Geometry: final body of the model. Coordinates: model frame, mm. Face numbers are marked on the shaded views. A direction names the side the tool comes from. Give positions to 0.01 mm unless a question says otherwise; leave off trailing zeros. Loops run counter-clockwise (first coordinate to the right, second up) from the corner with the lowest first, then second, coordinate; pieces in that order, holes last.
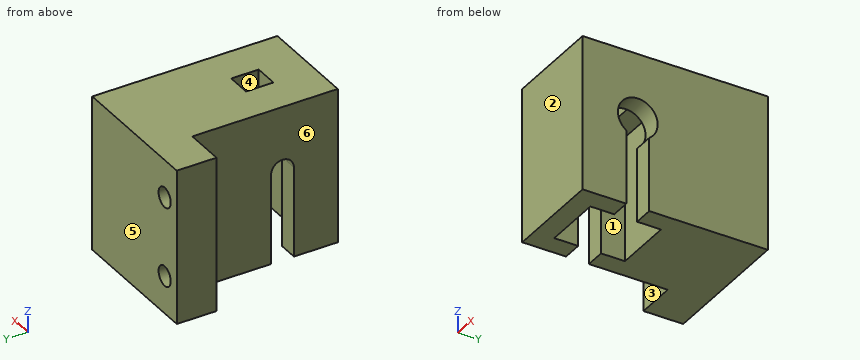
from build123d import *

# Parameters (mm, degrees)
SKETCH1_W           = 31.6
SKETCH1_H           = 35.300000012
SKETCH1_W_2         = 18.9
SKETCH1_H_2         = 22.600000012
BOSS_EXTRUDE1_DEPTH = 40
SKETCH2_W           = 31.6
SKETCH2_H           = 35.300000012
SKETCH2_W_2         = 18.9
SKETCH2_H_2         = 22.600000012
BOSS_EXTRUDE2_DEPTH = 9.525
SKETCH3_W           = 7.74908697
SKETCH3_H           = 8.788598638
CUT_EXTRUDE1_DEPTH  = 12.7
CUT_EXTRUDE2_DEPTH  = 31.75
SKETCH6_W           = 31.6
SKETCH6_H           = 49.525
BOSS_EXTRUDE3_DEPTH = 11.176
BOSS_EXTRUDE4_START = -44.45
SKETCH7_W           = 49.525
SKETCH7_H           = 6.35
BOSS_EXTRUDE4_DEPTH = 57.15
SKETCH8_R           = 3.175
CUT_EXTRUDE3_DEPTH  = 6.35
SKETCH9_W           = 12.85
SKETCH9_H           = 49.525
CUT_EXTRUDE4_DEPTH  = 6.35
SKETCH11_R          = 3.429
SKETCH11_W          = 12.85
SKETCH11_H          = 49.525
CUT_EXTRUDE5_DEPTH  = 6.35
SKETCH12_R          = 6.35
CUT_EXTRUDE6_DEPTH  = 6.35
SKETCH13_W          = 44.3
SKETCH13_H          = 49.525
SKETCH13_R          = 3.175
BOSS_EXTRUDE5_DEPTH = 12.7
SKETCH14_W          = 12.7
SKETCH14_H          = 49.525
SKETCH14_R          = 3.175
CUT_EXTRUDE7_DEPTH  = 6.35


with BuildPart() as part:
    # Sketch1 → Boss-Extrude1 (new body)
    with BuildSketch(Plane.XY):
        Rectangle(SKETCH1_W, SKETCH1_H)
        Rectangle(SKETCH1_W_2, SKETCH1_H_2, mode=Mode.SUBTRACT)
    extrude(amount=BOSS_EXTRUDE1_DEPTH)

    # Sketch2 → Boss-Extrude2 (add)
    # profile 1 of 2: a face of its own
    with BuildSketch(Plane.XY.offset(40)):
        Rectangle(SKETCH2_W, SKETCH2_H)
        Rectangle(SKETCH2_W_2, SKETCH2_H_2, mode=Mode.SUBTRACT)
    # profile 2 of 2: a face of its own
    with BuildSketch(Plane.XY.offset(40)):
        Rectangle(SKETCH2_W_2, SKETCH2_H_2)
    extrude(amount=BOSS_EXTRUDE2_DEPTH)

    # Sketch3 → Cut-Extrude1 (cut)
    with BuildSketch(Plane(origin=(0, 0, 40), x_dir=(-1, 0, 0), z_dir=(0, 0, -1))):
        Rectangle(SKETCH3_W, SKETCH3_H)
    extrude(amount=-CUT_EXTRUDE1_DEPTH, mode=Mode.SUBTRACT)

    # Sketch5 → Cut-Extrude2 (cut)
    with BuildSketch(Plane(origin=(15.8, 0, 0), x_dir=(0, 0, -1), z_dir=(1, 0, 0))):
        with BuildLine():
            Line((-28.827575985, 3.65), (0, 3.65))
            Line((0, 3.65), (0, -3.65))
            Line((0, -3.65), (-28.827575985, -3.65))
            ThreePointArc((-28.827575985, -3.65), (-32.477575985, 0), (-28.827575985, 3.65))
        make_face()
    extrude(amount=-CUT_EXTRUDE2_DEPTH, mode=Mode.SUBTRACT)

    # Sketch6 → Boss-Extrude3 (add)
    with BuildSketch(Plane(origin=(0, 17.650000006, 0), x_dir=(1, 0, 0), z_dir=(0, 1, 0))):
        with Locations((0, -24.7625)):
            Rectangle(SKETCH6_W, SKETCH6_H)
    extrude(amount=BOSS_EXTRUDE3_DEPTH)

    # Sketch7 → Boss-Extrude4 (add)
    with BuildSketch(Plane(origin=(15.8, 0, 0), x_dir=(0, 0, -1), z_dir=(1, 0, 0)).offset(BOSS_EXTRUDE4_START)):
        with Locations((-24.7625, 25.651000006)):
            Rectangle(SKETCH7_W, SKETCH7_H)
    boss_extrude4 = extrude(amount=BOSS_EXTRUDE4_DEPTH)

    # Sketch8 → Cut-Extrude3 (cut)
    with BuildSketch(Plane.XZ.offset(-22.476000006)):
        with Locations(Location((-22.225, 24.7625, 0), (0, 0, 270))):
            Circle(SKETCH8_R)
        with Locations(Location((22.15, 37.434572452, 0), (0, 0, 270))):
            Circle(SKETCH8_R)
        with Locations(Location((22.15, 12.034572452, 0), (0, 0, 270))):
            Circle(SKETCH8_R)
    extrude(amount=-CUT_EXTRUDE3_DEPTH, mode=Mode.SUBTRACT)

    # Sketch9 → Cut-Extrude4 (cut)
    with BuildSketch(Plane.XZ.offset(-22.476000006)):
        with Locations((-22.225, 24.7625)):
            Rectangle(SKETCH9_W, SKETCH9_H)
    extrude(amount=-CUT_EXTRUDE4_DEPTH, mode=Mode.SUBTRACT)

    # Mirror1: Boss-Extrude4 across plane
    add(boss_extrude4.mirror(Plane(origin=(0, 0, 0), x_dir=(0, 0, 1), z_dir=(1, 0, 0))))

    # Sketch11 → Cut-Extrude5 (cut)
    with BuildSketch(Plane(origin=(0, 28.826000006, 0), x_dir=(1, 0, 0), z_dir=(0, 1, 0))):
        with Locations(Location((-22.15, -37.4625, 0), (0, 0, 270))):
            Circle(SKETCH11_R)
        with Locations(Location((-22.15, -12.0625, 0), (0, 0, 270))):
            Circle(SKETCH11_R)
        with Locations((22.225, -24.7625)):
            Rectangle(SKETCH11_W, SKETCH11_H)
    extrude(amount=-CUT_EXTRUDE5_DEPTH, mode=Mode.SUBTRACT)

    # Sketch12 → Cut-Extrude6 (cut)
    with BuildSketch(Plane(origin=(15.8, 0, 0), x_dir=(0, 0, -1), z_dir=(1, 0, 0))):
        with Locations((-28.827575985, 0)):
            Circle(SKETCH12_R)
    extrude(amount=-CUT_EXTRUDE6_DEPTH, mode=Mode.SUBTRACT)

    # Sketch13 → Boss-Extrude5 (add)
    with BuildSketch(Plane(origin=(0, 28.826000006, 0), x_dir=(1, 0, 0), z_dir=(0, 1, 0))):
        with Locations((-6.35, -24.7625)):
            Rectangle(SKETCH13_W, SKETCH13_H)
        with Locations(Location((-22.15, -12.0625, 0), (0, 0, 270))):
            Circle(SKETCH13_R, mode=Mode.SUBTRACT)
        with Locations(Location((-22.15, -37.4625, 0), (0, 0, 270))):
            Circle(SKETCH13_R, mode=Mode.SUBTRACT)
    extrude(amount=BOSS_EXTRUDE5_DEPTH)

    # Sketch14 → Cut-Extrude7 (cut)
    with BuildSketch(Plane.XZ.offset(-22.476000006)):
        with Locations((-22.15, 24.7625)):
            Rectangle(SKETCH14_W, SKETCH14_H)
        with Locations(Location((-22.15, 37.4625, 0), (0, 0, 90))):
            Circle(SKETCH14_R, mode=Mode.SUBTRACT)
        with Locations(Location((-22.15, 12.0625, 0), (0, 0, 90))):
            Circle(SKETCH14_R, mode=Mode.SUBTRACT)
    extrude(amount=-CUT_EXTRUDE7_DEPTH, mode=Mode.SUBTRACT)


solid = part.part
Item 1: Ray query, probe 1 along Z at (x, y) = (-22, 37) (3 decimals); probe 2 along Y at (x, z) = (12.5, 22.5); probe 3 along X at (y, z) = (-0.5, 39). Return the intervals inside material, ascending.
Values follow:
probe 1: z = 0 to 8.891, 15.234 to 34.291, 40.634 to 49.525
probe 2: y = -17.65 to -3.65, 3.65 to 41.53
probe 3: x = -15.8 to -9.45, 9.45 to 15.8
Item 2: Section query D-D on x = -22.15. Return loops of the section in (y, z) (1 decimal).
Values follow:
outline: (28.8, 0) - (41.5, 0) - (41.5, 8.9) - (28.8, 8.9) - close; (28.8, 15.2) - (41.5, 15.2) - (41.5, 34.3) - (28.8, 34.3) - close; (28.8, 40.6) - (41.5, 40.6) - (41.5, 49.5) - (28.8, 49.5) - close
Item 3: Section query C-C on y = 0. Return loops of the section in (x, z) (3 decimals), plus the area to 3 significant figures.
Values follow:
outline: (-15.8, 32.478) - (-9.45, 32.478) - (-9.45, 40) - (-3.875, 40) - (-3.875, 49.525) - (-15.8, 49.525) - close; (3.875, 40) - (9.45, 40) - (9.45, 35.178) - (15.8, 35.178) - (15.8, 49.525) - (3.875, 49.525) - close
area: 306 mm2
Item 4: Section query A-A on z = 16.5. Return loops of the section in (x, y), plus the area to 3 significant figures.
Values follow:
outline: (-28.5, 28.83) - (-15.8, 28.83) - (-15.8, 3.65) - (-9.45, 3.65) - (-9.45, 11.3) - (9.45, 11.3) - (9.45, 3.65) - (15.8, 3.65) - (15.8, 41.53) - (-28.5, 41.53) - close; (-15.8, -17.65) - (15.8, -17.65) - (15.8, -3.65) - (9.45, -3.65) - (9.45, -11.3) - (-9.45, -11.3) - (-9.45, -3.65) - (-15.8, -3.65) - close
area: 1,510 mm2
Item 5: Pin query (flat end, axial travel): pin 1 (7.5 mm diameter, centred on y = 0, z = 28.83, fed in from +X); pin 2 (10 mm diameter, centred on x = -22, z = 33.5, fed in from -Y); pin 3 (9.5 mm diameter, centred on x = 3, y = 4, fed in from -Z); pin 4 (11.5 mm diameter, centred on y = 1, z = 10, fed in from +X). Return the tip coordinate at first contact, or that it passes through.
Values follow:
pin 1: stops at x = -9.45
pin 2: stops at y = 28.83
pin 3: stops at z = 40
pin 4: stops at x = 15.8
Item 6: Section query B-B on x = -1.5. Return loops of the section in (y, z) (3 decimals), plus the area to 3 significant figures.
Values follow:
outline: (-17.65, 0) - (-11.3, 0) - (-11.3, 40) - (-4.394, 40) - (-4.394, 49.525) - (-17.65, 49.525) - close; (4.394, 40) - (11.3, 40) - (11.3, 0) - (41.526, 0) - (41.526, 49.525) - (4.394, 49.525) - close
area: 1,940 mm2
Item 7: Draft query along X for the marked faces 4, 5 and 6. Return one class per face: +X half, -X half, draft (parallel to the pull), parting line (faces both ways), or undercut.
Values follow:
face 4: undercut
face 5: draft
face 6: -X half
Item 8: Set-up query: the marked faces 1, 2 and 3. Return all of +Z, -Z, +X, -X, +Y, -Y with unobstructed straight access to the full face (end or side cutting, diameter ignored); none if empty.
Values follow:
face 1: -Z
face 2: +Z, -Z, +X, -X, -Y
face 3: +Z, -Z, -X, -Y
